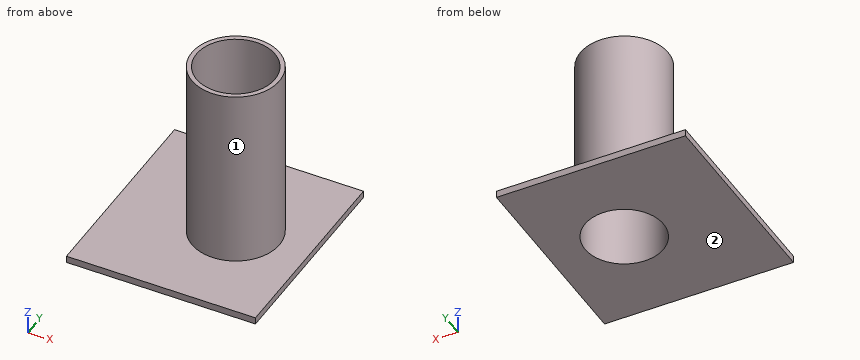
from build123d import *

# Parameters (mm, degrees)
BASE_R              = 17
BOSS_EXTRUDE1_DEPTH = 3
SKETCH1_R           = 19
SKETCH1_R_2         = 17
BOSS_EXTRUDE2_DEPTH = 80


with BuildPart() as part:
    # Base → Boss-Extrude1 (new body)
    with BuildSketch(Plane.XY):
        Polygon((-50, -44.45), (0, -44.45), (32, -44.45), (32, 44.45), (-50, 44.45), align=None)
        Circle(BASE_R, mode=Mode.SUBTRACT)
    extrude(amount=BOSS_EXTRUDE1_DEPTH)

    # Sketch1 → Boss-Extrude2 (add)
    with BuildSketch(Plane.XY.offset(3)):
        with Locations(Location((0, 0, 0), (0, 0, 180))):
            Circle(SKETCH1_R)
        Circle(SKETCH1_R_2, mode=Mode.SUBTRACT)
    extrude(amount=BOSS_EXTRUDE2_DEPTH)


solid = part.part
The listing builds one solid part. Answer for the finished solid, in the listing's coordinates (mm). Face numbers are marked on the shaded views. A direction names the side the tool comes from. Coordinates: 2 decimals unless noted, no trailing zeros. Order: outer loops, then holes, each group sorted by start corner. A loop starts at its lowest first (then second) coordinate and runs counter-clockwise, first axis right, second up. Notation, with made-up numbers: (5.5, 23) -> (62.5, 23) arc R17 ccw to (62.5, 34) -> close; hole circle Ø6 at (-30.75, 18). An arc over 180 degrees is marked (long way). Answer in a Markdown table with one row per item. Add a question column.
Item 1: Find section A-A (x = 0). Write down the section's boundary in (y, z), then the cut area to 3 significant figures.
Item 2: Find section B-B (y = 0). Write down the section's boundary in (x, z).
Item 3: Find section C-C (z = 76.5). Write down the section's boundary in (x, y).
Item 4: Find the intervals of material crossed by L1, parallel to Z at x = -18, y = 40; L2, parallel to Y at x = 0, z = 55; L3, parallel to Y at x = 5, z = 51, in increasing order. Write a range as from..to.
Item 5: Each of these flat-tipped pins is pushed along its axis until it touches: P1, Ø4, axis at y = -4, z = 68.5, coming from the +X side; P2, Ø8, axis at y = -5, z = 18, coming from the +X side; P3, Ø1.5, axis at x = 4, y = -29, coming from the +Z side. Where does it stop, or does it pass through?
Item 6: Find section D-D (x = -27.5). Write down the section's boundary in (y, z), then the cut area to 3 significant figures.
Item 7: Which of the six approach directions +Z, -Z, +X, -X, +Y, -Y give full straight-line access (tool end or side, diameter ignored) to the marked faces 1 and 2?
Result set:
| question | item | result |
|---|---|---|
| 1 | outline | (-44.45, 0) -> (-17, 0) -> (-17, 83) -> (-19, 83) -> (-19, 3) -> (-44.45, 3) -> close; (17, 0) -> (44.45, 0) -> (44.45, 3) -> (19, 3) -> (19, 83) -> (17, 83) -> close |
| 1 | area | 485 mm² |
| 2 | outline | (-50, 0) -> (-17, 0) -> (-17, 83) -> (-19, 83) -> (-19, 3) -> (-50, 3) -> close; (17, 0) -> (32, 0) -> (32, 3) -> (19, 3) -> (19, 83) -> (17, 83) -> close |
| 3 | outline | circle Ø38 at (0, 0); hole circle Ø34 at (0, 0) |
| 4 | L1 | z = 0..3 |
| 4 | L2 | y = -19..-17, 17..19 |
| 4 | L3 | y = -18.33..-16.25, 16.25..18.33 |
| 5 | P1 | stops at x = 18.89 |
| 5 | P2 | stops at x = 18.97 |
| 5 | P3 | stops at z = 3 |
| 6 | outline | (-44.45, 0) -> (44.45, 0) -> (44.45, 3) -> (-44.45, 3) -> close |
| 6 | area | 267 mm² |
| 7 | face 1 | +Z |
| 7 | face 2 | -Z, +X, -X, +Y, -Y |
